from build123d import *

# Parameters (mm, degrees)
F1_DEPTH = 25.4
F2_DEPTH = 27.94


with BuildPart() as f1:
    # F0 (on Front) → F1 (new body)
    with BuildSketch(Plane.XZ):
        Polygon((0, 26.830262), (0, 37.234288), (-5.556555, 46.435609), (-2.240721, 46.435609), (-2.240721, 53.097513), (-16.439889, 53.097513), (-16.439889, 46.435609), (-12.975313, 46.435609), (-24.338637, 28.06516), (-27.128741, 28.06516), (-27.128741, 21.727359), (-12.54946, 21.727359), (-12.54946, 28.06516), (-16.439889, 28.06516), (-9.336166, 39.656349), (-5.951528, 33.498235), (-8.177853, 33.498235), (-8.177853, 26.830262), align=None)
    extrude(amount=F1_DEPTH)

    # F0 (on Front) → F2 (join)
    with BuildSketch(Plane.XZ):
        Polygon((0, 37.234288), (0, 39.675493), (-3.814953, 45.588929), (-0.95885, 45.588929), (-0.95885, 54.082506), (-17.337842, 54.082506), (-17.337842, 45.48464), (-14.827147, 45.48464), (-24.975492, 29.078379), (-28.187823, 29.078379), (-28.187823, 20.709392), (-11.463354, 20.709392), (-11.463354, 29.128009), (-14.395286, 29.128009), (-9.349254, 37.361652), (-7.894423, 34.714688), (-9.349254, 34.714688), (-9.349254, 25.930258), (0, 25.930258), (0, 26.830262), (-8.177853, 26.830262), (-8.177853, 33.498235), (-5.951528, 33.498235), (-9.336166, 39.656349), (-16.439889, 28.06516), (-12.54946, 28.06516), (-12.54946, 21.727359), (-27.128741, 21.727359), (-27.128741, 28.06516), (-24.338637, 28.06516), (-12.975313, 46.435609), (-16.439889, 46.435609), (-16.439889, 53.097513), (-2.240721, 53.097513), (-2.240721, 46.435609), (-5.556555, 46.435609), align=None)
    extrude(amount=F2_DEPTH)

    # F3: F1 across face


with BuildPart() as f1_1:
    add(f1.part)
    add(f1.part.mirror(Plane(origin=(0, -13.031526, 32.859819), x_dir=(0, 1, 0), z_dir=(1, 0, 0))))


solid = f1_1.part
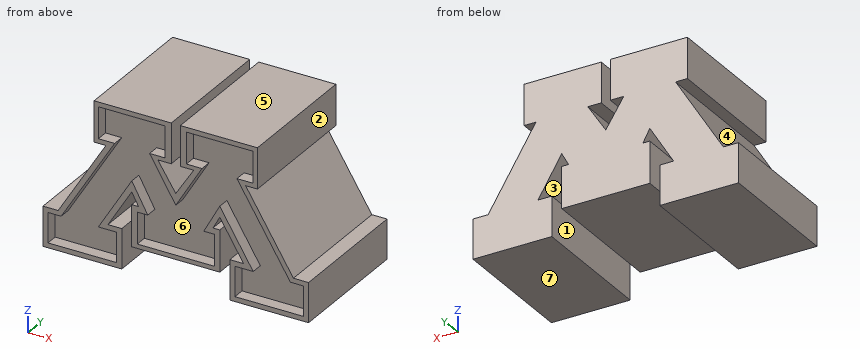
Could you check a few things on this model? Use its own coordinates, in mm. Face numbers are marked on the shaded views. A direction names the side the tool comes from. Round coordinates to 2 decimals unless told otherwise and drop trailing zeros. Order: outer loops, then holes, each group sorted by start corner. A loop starts at its lowest first (then second) coordinate and runs counter-clockwise, first axis right, second up. Notation, with made-up numbers: M 70.25,29 L 104.25,29 A32 cw 104.25,64 Z; hole C 74.5,24.25 d3. An arc over 180 degrees is marked long. One line per item, written item: value.
(1) I'm going to push flat-ended pins straight in: P1, Ø7, axis at y = -7.5, z = 50, coming from the +X side; P2, Ø5.5, axis at x = -4, y = -16, coming from the -Z side; P3, Ø2, axis at y = -19.5, z = 33, coming from the +X side. Where does each tip first touch, or does it pass through?
Ans:
P1: stops at x = 17.34
P2: stops at z = 25.93
P3: stops at x = 23.17
(2) Which directions (+Z, -Z, +X, -X, +Y, -Y) give clear straight access to the entire face, cutting with the end or side of a thin tool? Please do the marked faces 1, 2, 3 and 4.
Ans:
face 1: -Z, +Y, -Y
face 2: +Z, +X, +Y, -Y
face 3: +Y, -Y
face 4: -X, +Y, -Y
(3) If we mould it in two halves opening along Z, with no side actions, what happens to the marked faces 5, 6 and 7? For each: released by +Z, released by -Z, zero draft, split by the parting line, or undercut.
Ans:
face 5: released by +Z
face 6: undercut
face 7: released by -Z
(4) Imagine slicing it at B-B (z = 36.5). Write out the boundary of the cut face in (x, y).
Ans:
outline: M -20.38,-27.94 L -19.12,-27.94 L -19.12,-25.4 L -11.27,-25.4 L -11.27,-27.94 L -9.88,-27.94 L -9.88,0 L -20.38,0 Z; M -8.88,-27.94 L -7.6,-27.94 L -7.6,-25.4 L 7.6,-25.4 L 7.6,-27.94 L 8.88,-27.94 L 8.88,0 L -8.88,0 Z; M 9.88,-27.94 L 11.27,-27.94 L 11.27,-25.4 L 19.12,-25.4 L 19.12,-27.94 L 20.38,-27.94 L 20.38,0 L 9.88,0 Z
(5) Imagine slicing it at A-A (z = 49). Write out the boundary of the cut face in (x, y).
Ans:
outline: M -17.34,-27.94 L -16.44,-27.94 L -16.44,-25.4 L -2.24,-25.4 L -2.24,-27.94 L -0.96,-27.94 L -0.96,0 L -17.34,0 Z; M 0.96,-27.94 L 2.24,-27.94 L 2.24,-25.4 L 16.44,-25.4 L 16.44,-27.94 L 17.34,-27.94 L 17.34,0 L 0.96,0 Z
(6) I need wall thicknesses on line 1 along X through (y, z) = (-4, 27.5); line 2 along X through (y, z) = (-21.75, 50.5); line 3 along X through (y, z) = (-1.75, 35). Which ranges of each line are inside material? Lowest first, please. Write a range as from..to.
Ans:
line 1: x = -28.19..-11.46, -9.35..9.35, 11.46..28.19
line 2: x = -17.34..-0.96, 0.96..17.34
line 3: x = -21.31..-10.8, -8.05..8.05, 10.8..21.31
(7) Imagine slicing it at D-D (x = -7). Write out the boundary of the cut face in (y, z), and give its area (3 significant figures).
Ans:
outline: M -27.94,25.93 L 0,25.93 L 0,54.08 L -27.94,54.08 L -27.94,53.1 L -25.4,53.1 L -25.4,35.41 L -27.94,35.41 L -27.94,33.5 L -25.4,33.5 L -25.4,26.83 L -27.94,26.83 Z
area: 725 mm^2
